```python
from build123d import *

# Parameters (mm, degrees)
ESQUISSE1_R                  = 2.5
BOSS_EXTRU_1_DEPTH           = 7.5
ESQUISSE2_R                  = 3.5
BOSS_EXTRU_2_DEPTH           = 29.5
ESQUISSE3_R                  = 3
BOSS_EXTRU_3_DEPTH           = 0.75
ESQUISSE4_R                  = 3.5
BOSS_EXTRU_4_DEPTH           = 2
ESQUISSE5_R                  = 3
BOSS_EXTRU_5_DEPTH           = 0.75
ESQUISSE6_R                  = 3.5
BOSS_EXTRU_6_DEPTH           = 2.5
ESQUISSE7_R                  = 3
BOSS_EXTRU_7_DEPTH           = 0.5
ESQUISSE8_R                  = 3.5
BOSS_EXTRU_8_DEPTH           = 9
CHANFREIN2_SIZE              = 0.5
ENL_V_MAT_EXTRU_1_DEPTH      = 53.732817107
ENL_V_MAT_EXTRU_1_DEPTH_BACK = 53.732817107
ESQUISSE9_R                  = 1


with BuildPart() as part:
    # Esquisse1 → Boss.-Extru.1 (new body)
    with BuildSketch(Plane.XY):
        Circle(ESQUISSE1_R)
    extrude(amount=BOSS_EXTRU_1_DEPTH)

    # Esquisse2 → Boss.-Extru.2 (add)
    with BuildSketch(Plane.XY.offset(7.5)):
        Circle(ESQUISSE2_R)
    extrude(amount=BOSS_EXTRU_2_DEPTH)

    # Esquisse3 → Boss.-Extru.3 (add)
    with BuildSketch(Plane.XY.offset(37)):
        Circle(ESQUISSE3_R)
    extrude(amount=BOSS_EXTRU_3_DEPTH)

    # Esquisse4 → Boss.-Extru.4 (add)
    with BuildSketch(Plane.XY.offset(37.75)):
        Circle(ESQUISSE4_R)
    extrude(amount=BOSS_EXTRU_4_DEPTH)

    # Esquisse5 → Boss.-Extru.5 (add)
    with BuildSketch(Plane.XY.offset(39.75)):
        Circle(ESQUISSE5_R)
    extrude(amount=BOSS_EXTRU_5_DEPTH)

    # Esquisse6 → Boss.-Extru.6 (add)
    with BuildSketch(Plane.XY.offset(40.5)):
        Circle(ESQUISSE6_R)
    extrude(amount=BOSS_EXTRU_6_DEPTH)

    # Esquisse7 → Boss.-Extru.7 (add)
    with BuildSketch(Plane.XY.offset(43)):
        Circle(ESQUISSE7_R)
    extrude(amount=BOSS_EXTRU_7_DEPTH)

    # Esquisse8 → Boss.-Extru.8 (add)
    with BuildSketch(Plane.XY.offset(43.5)):
        Circle(ESQUISSE8_R)
    extrude(amount=BOSS_EXTRU_8_DEPTH)

    # Chanfrein2
    chanfrein2_edges = [part.edges().sort_by_distance(p)[0] for p in [
        (-2.5, 0, 0),
        (-3.5, 0, 52.5),
    ]]
    chamfer(chanfrein2_edges, length=CHANFREIN2_SIZE)

    # Esquisse9 → Enlèv. mat.-Extru.1 (cut, two sides: drawn at the far end of the back side and taken through both)
    with BuildSketch(Plane(origin=(0, 0, 0), x_dir=(1, 0, 0), z_dir=(0, 1, 0)).offset(-ENL_V_MAT_EXTRU_1_DEPTH_BACK)):
        with Locations(Location((0, -17.5, 0), (0, 0, 270))):
            Circle(ESQUISSE9_R)
    extrude(amount=ENL_V_MAT_EXTRU_1_DEPTH + ENL_V_MAT_EXTRU_1_DEPTH_BACK, mode=Mode.SUBTRACT)


solid = part.part
```
Part model, mm, in its own coordinate system. A direction names the side the tool comes from. Coordinates: 2 decimals unless noted, no trailing zeros. Loops run counter-clockwise (first coordinate to the right, second up) from the corner with the lowest first, then second, coordinate; pieces in that order, holes last. Notation, with made-up numbers: (68.25, 26) - (98.25, 26) arc R26 cw to (98.25, 55) - close; hole circle Ø4 at (31, 69.25). An arc over 180 degrees is marked (long way). Write item = value, one per line. Start each with the question number.
Item 1: Flat gauge pin, fed straight in: pin 1 Ø1.8 at (x, z) = (0, 17.5) entering from -Y. Where does the tip first touch, or does it go through?
Item 2: 3-axis set-ups, long thin cutter, end or side, ignore diameter. For faces 5 (the flat face through (3, 1, 40.5)), 6 (the flat face through (2, -2, 7.5)), 7 (the cylindrical face through (-0.383, -0.049, 18.424)): which of +Z, -Z, +X, -X, +Y, -Y reach the whole face in a straight line?
Item 3: Wall check: L1, parallel to Z at x = 0, y = -1; L2, parallel to Z at x = 2.5, y = -2.25; L3, parallel to Z at x = 2.5, y = 1.75. Give the ranges that are in metal, low to high. Write a range as from..to.
Item 4: Cut at A-A, the plane z = 26.5. Give the cut face in (x, y).
Item 5: Mould opens along Z. For faces 1 (the flat face through (3, 1, 39.75)), 2 (the flat face through (0, 0, 0)), 3 (the cylindrical face through (-0.54, -2.44, 3.95)), 4 (the flat face through (3, 1, 37.75)) say: released by +Z, released by -Z, zero draft, split by the parting line, or undercut.
Item 6: Cut at B-B, the plane z = 17.5. Give the cut face in (x, y), and give its area (3 significant figures).
The answers:
q1.pin_1 = through
q2.face_5 = none
q2.face_6 = -Z
q2.face_7 = +Y, -Y
q3.L1 = 0..16.5, 18.5..52.5
q3.L2 = 7.5..37, 37.75..39.75, 40.5..43, 43.5..52.14
q3.L3 = 7.5..37, 37.75..39.75, 40.5..43, 43.5..52.45
q4.outline = circle Ø7 at (0, 0)
q5.face_1 = undercut
q5.face_2 = released by -Z
q5.face_3 = zero draft
q5.face_4 = undercut
q6.outline = (-1, -3.35) - (-1, 3.35) arc R3.5 ccw to start; (1, -3.35) arc R3.5 ccw to (1, 3.35) - close
q6.area = 24.7 mm2
